```python
from build123d import *

# Parameters (mm, degrees)
F0_W     = 152.4
F0_H     = 76.2
F1_DEPTH = 6.35
F2_W     = 138.938
F2_H     = 6.35
F3_DEPTH = 69.85
F4_R     = 19.05
F4_R_2   = 7.9375
F5_DEPTH = 50.8
F6_R     = 7.9375
F7_DEPTH = 7.62
F8_SIZE  = 5.08
F9_SIZE  = 5.08


with BuildPart() as f1:
    # F0 (on Top) → F1 (new body)
    with BuildSketch(Plane.XY):
        Rectangle(F0_W, F0_H)
    extrude(amount=F1_DEPTH)

    # F2 (on face) → F3 (join)
    with BuildSketch(Plane.XY.offset(6.35)):
        Polygon((-69.088, 38.1), (-76.2, 38.1), (-76.2, -38.1), (-69.088, -38.1), (-69.088, -31.75), (-69.088, 31.75), align=None)
        Polygon((76.2, 38.1), (-69.088, 38.1), (-69.088, 31.75), (69.85, 31.75), (76.2, 31.75), align=None)
        with Locations((0.381, -34.925)):
            Rectangle(F2_W, F2_H)
        Polygon((76.2, 31.75), (69.85, 31.75), (69.85, -31.75), (69.85, -38.1), (76.2, -38.1), align=None)
    extrude(amount=F3_DEPTH)

    # F4 (on face) → F5 (join)
    with BuildSketch(Plane(origin=(-76.2, 0, 0), x_dir=(0, -1, 0), z_dir=(-1, 0, 0))):
        with Locations((0, 38.1)):
            Circle(F4_R)
        with Locations((0, 38.1)):
            Circle(F4_R_2, mode=Mode.SUBTRACT)
    extrude(amount=F5_DEPTH)

    # F6 (on face) → F7 (cut)
    with BuildSketch(Plane(origin=(-76.2, 0, 0), x_dir=(0, -1, 0), z_dir=(-1, 0, 0))):
        with Locations((0, 38.1)):
            Circle(F6_R)
    extrude(amount=-F7_DEPTH, mode=Mode.SUBTRACT)

    # F8
    f8_edges = [f1.edges().sort_by_distance(p)[0] for p in [
        (-69.088, 7.9375, 38.1),
    ]]
    chamfer(f8_edges, length=F8_SIZE)

    # F9
    f9_edges = [f1.edges().sort_by_distance(p)[0] for p in [
        (-127, 7.9375, 38.1),
    ]]
    chamfer(f9_edges, length=F9_SIZE)


solid = f1.part
```
Model file for the job. Use its own axes, mm. A direction names the side the tool comes from. Coordinates: 2 decimals unless noted, no trailing zeros. Order: outer loops, then holes, each group sorted by start corner. A loop starts at its lowest first (then second) coordinate and runs counter-clockwise, first axis right, second up. Notation, with made-up numbers: (88, 57) -> (126, 57) arc R33 ccw to (126, 96) -> close; hole circle Ø11 at (58, -16.75). An arc over 180 degrees is marked (long way). Answer as a JSON object with one key per item and string values. Group by question number.
1) Which spindle directions (+Z, -Z, +X, -X, +Y, -Y) get a long thin tool onto all of the face, cutting with end or side? Do faces 5 (the face through (69.85, 0, 41)), 6 (the face through (-101.244, 4.13, 19.503)), 7 (the face through (-73.92, -4.4, 45)). Say none if no direction does.
2) Cut at B-B, the plane z = 15. Write the cut outline in (x, y), then the cut area to 3 significant figures.
3) Cut at A-A, the plane y = 0. Write the cut outline in (x, z).
4) Cut at D-D, the plane z = 38.1. Write the cut outline in (x, y), then the cut area to 3 significant figures.
5) Cut at C-C, the plane y = -26. Write the cut outline in (x, z).
6) Drill centre lines: L1, parallel to X at y = 6, z = 58.5; L2, parallel to Y at x = -57.5, z = 10.5; L3, parallel to X at y = -17.5, z = 33.5. Where is each one in solid material? Low to high.
7) Pull direction Y, two halves, no side cores. Call faces 1 (the face through (-1, -38.1, 38)), 2 (the face through (-1, 0, 6.35)), 3 (the face through (1, 38.1, 38)), 4 (the face through (-1, 1, 0)): +Y half, -Y half, draft (parallel to the pull), parting line (faces both ways), or undercut.
8) Flat gauge pins, fed straight in: pin 1 (8 mm diameter, centred on x = -103, y = 16, fed in from -Z); pin 2 (8 mm diameter, centred on x = -104, z = 33, fed in from -Y); pin 3 (4 mm diameter, centred on y = -25.5, z = 24, fed in from -X). Where does each tip first touch, or does it go through?
Check values:
{
 "1": {"face 5": "+Z", "face 6": "-X", "face 7": "none"},
 "2": {"outline": "(-76.2, -38.1) -> (76.2, -38.1) -> (76.2, 38.1) -> (-76.2, 38.1) -> close; hole (-69.09, -31.75) -> (69.85, -31.75) -> (69.85, 31.75) -> (-69.09, 31.75) -> close", "area": "2,790 mm²"},
 "3": {"outline": "(-127, 19.05) -> (-76.2, 19.05) -> (-76.2, 0) -> (76.2, 0) -> (76.2, 76.2) -> (69.85, 76.2) -> (69.85, 6.35) -> (-69.09, 6.35) -> (-69.09, 25.08) -> (-74.17, 30.16) -> (-121.92, 30.16) -> (-127, 25.08) -> close; (-127, 51.12) -> (-121.92, 46.04) -> (-74.17, 46.04) -> (-69.09, 51.12) -> (-69.09, 76.2) -> (-76.2, 76.2) -> (-76.2, 57.15) -> (-127, 57.15) -> close"},
 "4": {"outline": "(-127, -19.05) -> (-76.2, -19.05) -> (-76.2, -38.1) -> (76.2, -38.1) -> (76.2, 38.1) -> (-76.2, 38.1) -> (-76.2, 19.05) -> (-127, 19.05) -> (-127, 13.02) -> (-121.92, 7.94) -> (-74.17, 7.94) -> (-69.09, 13.02) -> (-69.09, 31.75) -> (69.85, 31.75) -> (69.85, -31.75) -> (-69.09, -31.75) -> (-69.09, -13.02) -> (-74.17, -7.94) -> (-121.92, -7.94) -> (-127, -13.02) -> close", "area": "3,750 mm²"},
 "5": {"outline": "(-76.2, 0) -> (76.2, 0) -> (76.2, 76.2) -> (69.85, 76.2) -> (69.85, 6.35) -> (-69.09, 6.35) -> (-69.09, 76.2) -> (-76.2, 76.2) -> close"},
 "6": {"L1": "x = -76.2 to -69.09, 69.85 to 76.2", "L2": "y = -38.1 to -31.75, 31.75 to 38.1", "L3": "x = -127 to -69.09, 69.85 to 76.2"},
 "7": {"face 1": "-Y half", "face 2": "undercut", "face 3": "+Y half", "face 4": "draft"},
 "8": {"pin 1": "stops at z = 23.3", "pin 2": "stops at y = -19.02", "pin 3": "stops at x = -76.2"}
}
